Work out the finished part from the listing and answer in its coordinate system (mm). Face numbers are marked on the shaded views. A direction names the side the tool comes from. Coordinates: 2 decimals unless noted, no trailing zeros. Order: outer loops, then holes, each group sorted by start corner. A loop starts at its lowest first (then second) coordinate and runs counter-clockwise, first axis right, second up. Notation, with made-up numbers: M -27,-0.5 L -3,-0.5 A15 cw -3,12.5 Z; hole C -38.75,21.25 d6. An arc over 180 degrees is marked long. Use a Markdown table: item, result.
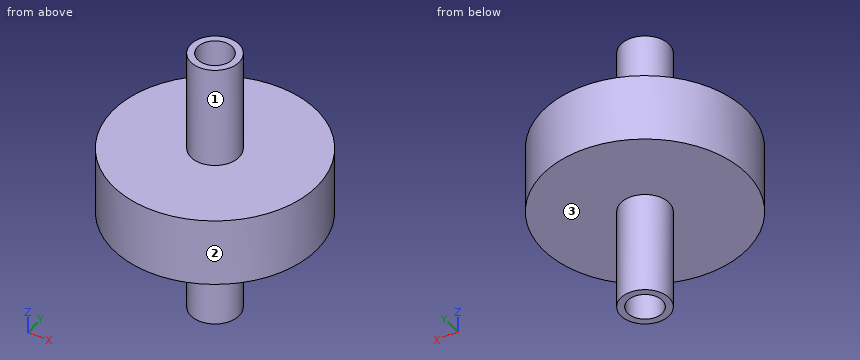
from build123d import *

# Parameters (mm, degrees)
SKETCH3_R                = 15
BOSS_EXTRUDE1_DEPTH      = 10
SKETCH4_R                = 3.55
SKETCH4_R_2              = 2.55
BOSS_EXTRUDE2_DEPTH      = 15
BOSS_EXTRUDE2_DEPTH_BACK = 25
SKETCH9_R                = 2.55
CUT_EXTRUDE1_DEPTH       = 26


with BuildPart() as part:
    # Sketch3 → Boss-Extrude1 (new body)
    with BuildSketch(Plane.XY):
        Circle(SKETCH3_R)
    extrude(amount=BOSS_EXTRUDE1_DEPTH)

    # Sketch4 → Boss-Extrude2 (add, two sides)
    with BuildSketch(Plane.XY.offset(10)) as boss_extrude2_sk:
        Circle(SKETCH4_R)
        Circle(SKETCH4_R_2, mode=Mode.SUBTRACT)
    extrude(amount=BOSS_EXTRUDE2_DEPTH)
    extrude(boss_extrude2_sk.sketch, amount=-BOSS_EXTRUDE2_DEPTH_BACK)

    # Sketch9 → Cut-Extrude1 (cut, through all)
    with BuildSketch(Plane.XY.offset(10)):
        Circle(SKETCH9_R)
    extrude(amount=-CUT_EXTRUDE1_DEPTH, mode=Mode.SUBTRACT)


solid = part.part
1. Flat-ended cylindrical pins translate along their axes: P1, Ø10, axis at x = 4, y = -11.5, coming from the -Z side; P2, Ø3, axis at y = -9, z = 2, coming from the +X side; P3, Ø3, axis at y = 8.5, z = 13, coming from the -X side (1 decimal); P4, Ø10, axis at y = 6, z = 7.5, coming from the -X side. Find the tip coordinate at first contact, or state that the pin passes through.
Answers below:
| item | result |
|---|---|
| P1 | z = 0 |
| P2 | x = 12.99 |
| P3 | through |
| P4 | x = -14.97 |
2. Section C-C on z = 13.5 is taken. Determine the outline of the cut face in (x, y).
Answers below:
| item | result |
|---|---|
| outline | C 0,0 d7.1; hole C 0,0 d5.1 |
3. Section D-D on z = 2 is taken. Determine the outline of the cut face in (x, y).
Answers below:
| item | result |
|---|---|
| outline | C 0,0 d30; hole C 0,0 d5.1 |
4. Find the intervals of material crossed by probe 1 along Y at (x, z) = (0.25, 5); probe 2 along Y at (x, z) = (0, -4.25); probe 3 along Z at (x, y) = (-7.75, -0.5), in increasing order.
Answers below:
| item | result |
|---|---|
| probe 1 | -15 to -2.54, 2.54 to 15 |
| probe 2 | -3.55 to -2.55, 2.55 to 3.55 |
| probe 3 | 0 to 10 |
5. Section A-A on x = 0 is taken. Determine the outline of the cut face in (y, z), then the cut area to 3 significant figures.
Answers below:
| item | result |
|---|---|
| outline | M -15,0 L -3.55,0 L -3.55,-15 L -2.55,-15 L -2.55,25 L -3.55,25 L -3.55,10 L -15,10 Z; M 2.55,-15 L 3.55,-15 L 3.55,0 L 15,0 L 15,10 L 3.55,10 L 3.55,25 L 2.55,25 Z |
| area | 309 mm² |
6. For the marked faces 1, 2 and 3, determine the directions among +Z, -Z, +X, -X, +Y, -Y from which every point of the face is accessible in a straight line to the end or side of a thin tool.
Answers below:
| item | result |
|---|---|
| face 1 | +Z |
| face 2 | +Z, -Z |
| face 3 | -Z |
